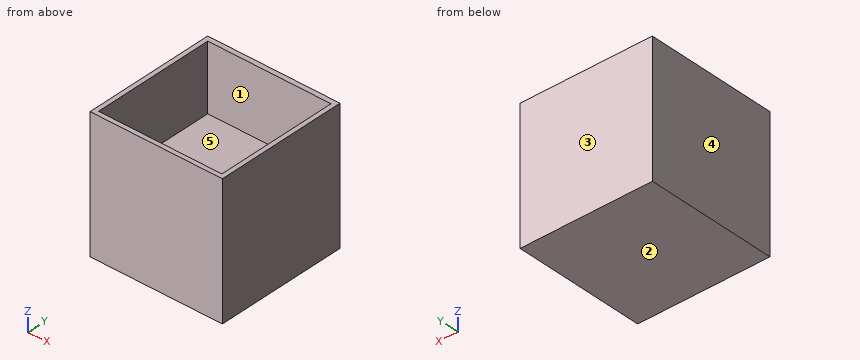
from build123d import *

# Parameters (mm, degrees)
F0_W     = 50.8
F0_H     = 50.8
F1_DEPTH = 50.8
F2_W     = 47.356754
F2_H     = 47.165799
F3_DEPTH = 25.4


with BuildPart() as f1:
    # F0 (on Front) → F1 (new body)
    with BuildSketch(Plane.XZ):
        with Locations((-25.4, 25.4)):
            Rectangle(F0_W, F0_H)
    extrude(amount=F1_DEPTH)

    # F2 (on face) → F3 (cut)
    with BuildSketch(Plane.XY.offset(50.8)):
        with Locations((-25.396969, -25.492446)):
            Rectangle(F2_W, F2_H)
    extrude(amount=-F3_DEPTH, mode=Mode.SUBTRACT)


solid = f1.part
Here's how the part is built. I have some questions about the finished solid (model axes, mm). Face numbers are marked on the shaded views. A direction names the side the tool comes from. Round coordinates to 2 decimals unless told otherwise and drop trailing zeros. Order: outer loops, then holes, each group sorted by start corner. A loop starts at its lowest first (then second) coordinate and runs counter-clockwise, first axis right, second up. Notation, with made-up numbers: M 38,24.25 L 60,24.25 A31 cw 60,54.25 Z; hole C -23.75,10.5 d4. An arc over 180 degrees is marked long. Return JSON: item names as keys, results as strings. Group by question number.
1. If we section it at B-B on x = -47: List the corners of the cut face in (y, z) for me, then the cut area to 3 significant figures.
2. If we section it at A-A on y = -45.5: List the corners of the cut face in (x, z) for me.
3. I'm going to push a flat-ended pin straight in: pin 1 Ø6 at (x, y) = (-32.5, -11) entering from +Z. Where does the tip first touch, or does it pass through?
4. If we section it at C-C on z = 40.5: List the corners of the cut face in (x, y) for me, then the cut area to 3 significant figures.
5. If we mould it in two halves opening along Y, with no side actions, what happens to the marked faces 3, 4 and 5? For each: pulls with the +Y half, pulls with the -Y half, needs draft (parallel to the pull), parting line crosses it, or undercut.
6. Please list where these lines run through material, in increasing order: probe 1 along Y at (x, z) = (-31, 36.5); probe 2 along X at (y, z) = (-40, 41.5); probe 3 along Z at (x, y) = (-30, -45).
7. On a 3-axis mill with a long thin cutter (end or side, diameter ignored), from which of +Z, -Z, +X, -X, +Y, -Y can I reach the whole of each face in a straight line? I mean the marked faces 1 and 2. Say none if no direction works.
Reply:
{
 "1": {"outline": "M -50.8,0 L 0,0 L 0,50.8 L -1.91,50.8 L -1.91,25.4 L -49.08,25.4 L -49.08,50.8 L -50.8,50.8 Z", "area": "1,380 mm^2"},
 "2": {"outline": "M -50.8,0 L 0,0 L 0,50.8 L -1.72,50.8 L -1.72,25.4 L -49.08,25.4 L -49.08,50.8 L -50.8,50.8 Z"},
 "3": {"pin 1": "z = 25.4"},
 "4": {"outline": "M -50.8,-50.8 L 0,-50.8 L 0,0 L -50.8,0 Z; hole M -49.08,-49.08 L -1.72,-49.08 L -1.72,-1.91 L -49.08,-1.91 Z", "area": "347 mm^2"},
 "5": {"face 3": "pulls with the +Y half", "face 4": "needs draft", "face 5": "undercut"},
 "6": {"probe 1": "-50.8 to -49.08, -1.91 to 0", "probe 2": "-50.8 to -49.08, -1.72 to 0", "probe 3": "0 to 25.4"},
 "7": {"face 1": "+Z", "face 2": "-Z, +X, -X, +Y, -Y"}
}
